For this review, take the finished solid that the model builds, in its own axes (mm). Face numbers are marked on the shaded views. A direction names the side the tool comes from. Coordinates: 2 decimals unless noted, no trailing zeros. Order: outer loops, then holes, each group sorted by start corner. A loop starts at its lowest first (then second) coordinate and runs counter-clockwise, first axis right, second up.
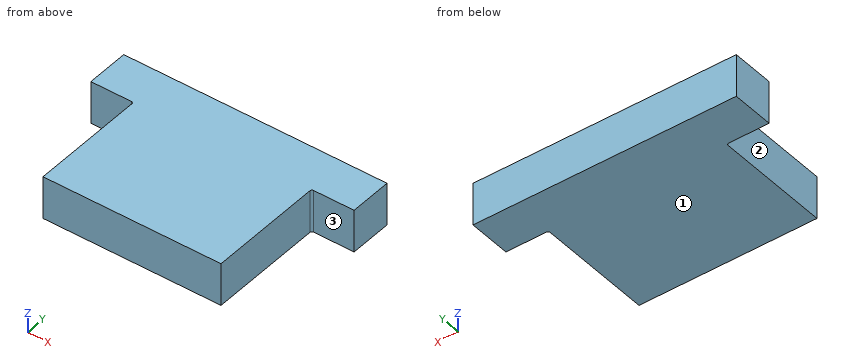
Autodesk Inventor part; units mm, degrees
ref_plane "YZ Plane" through (0, 0, 0) normal (1, 0, 0) x (0, 1, 0)
ref_plane "XZ Plane" through (0, 0, 0) normal (0, 1, 0) x (-1, 0, 0)
ref_plane "XY Plane" through (0, 0, 0) normal (0, 0, 1) x (1, 0, 0)
sketch "Sketch1" plane through (0, 0, 0) normal (0, 0, 1) x (1, 0, 0)
  line L0 (4.175, -3.75) -> (-4.175, -3.75)
  line L1 (-4.175, -3.75) -> (-4.175, 3.75)
  line L2 (-4.175, 3.75) -> (4.175, 3.75)
  line L3 (4.175, 3.75) -> (4.175, -3.75)
  line L4 (4.175, -3.75) -> (-4.175, 3.75) construction
  line L5 (-4.175, -3.75) -> (4.175, 3.75) construction
  point P0 (0, 0)
  dimension "d0" = 8.35
  dimension "d1" = 7.5
extrude "Extrusion1" add sketch "Sketch1" along normal mid plane 2
sketch "Sketch2" plane through (4.175, -3.75, 1) normal (1, 0, 0) x (0, 0, -1)
  line L0 (2, 7.5) -> (0, 7.5)
  line L1 (2, 7.5) -> (0, 7.5)
  line L2 (0, 7.5) -> (0, 5.5)
  line L3 (0, 5.5) -> (2, 5.5)
  line L4 (2, 5.5) -> (2, 7.5)
  point P0 (1, 3.75)
  dimension "d4" = 2
  dimension "d5" = 2
extrude "Extrusion2" add sketch "Sketch2" along normal blind 2
sketch "Sketch3" plane through (-4.175, -3.75, 1) normal (-1, 0, 0) x (0, 0, 1)
  line L0 (-2, 7.5) -> (0, 7.5)
  line L1 (0, 7.5) -> (0, 0)
  line L2 (-2, 7.5) -> (0, 7.5)
  line L3 (0, 7.5) -> (0, 5.5)
  line L4 (0, 5.5) -> (-2, 5.5)
  line L5 (-2, 5.5) -> (-2, 7.5)
  point P0 (-1, 3.75)
  dimension "d8" = 2
extrude "Extrusion3" add sketch "Sketch3" along normal blind 2
fillet "Fillet1" radius 0.1 2 edges at (4.175, 1.75, 0) (-4.175, 1.75, 0)
properties part number "Tapa_2_TFM"
1. Clearance check with flat-ended pins moving along their axes: pin 1 Ø0.9 at (x, z) = (5.5, 0) entering from -Y; pin 2 Ø1 at (y, z) = (-1, 0) entering from -X (3 decimals). State where each tip first meets the part, or that it passes through.
Answer below:
pin 1: stops at y = 1.75
pin 2: stops at x = -4.175
2. Machinability: for the marked faces 1, 2 and 3, which of the approach directions +Z, -Z, +X, -X, +Y, -Y give a long, thin tool a straight path to every point of the face, cutting with its end or side? Answer none if there is none.
Answer below:
face 1: -Z, +X, -X, +Y, -Y
face 2: +Z, -Z, -X, -Y
face 3: +Z, -Z, +X, -Y
3. To check wall thickness, follow L1, parallel to Y at x = 4.5, z = 0.5; L2, parallel to X at y = -2.5, z = -0.6 (3 decimals). State the ranges of each line that lie inside material, in increasing order.
Answer below:
L1: y = 1.75 to 3.75
L2: x = -4.175 to 4.175
4. Take a section at A-A, the plane z = 0.75. Give the boundary of the cut face in (x, y) (3 decimals), plus the area to 3 significant figures.
Answer below:
outline: (-6.175, 1.75) - (-4.275, 1.75) arc R0.1 cw to (-4.175, 1.65) - (-4.175, -3.75) - (4.175, -3.75) - (4.175, 1.65) arc R0.1 cw to (4.275, 1.75) - (6.175, 1.75) - (6.175, 3.75) - (-6.175, 3.75) - close
area: 70.6 mm2
5. Take a section at C-C, the plane y = 0.75. Give the boundary of the cut face in (x, z) (3 decimals).
Answer below:
outline: (-4.175, -1) - (4.175, -1) - (4.175, 1) - (-4.175, 1) - close
6. Take a section at B-B, the plane x = 5. Give the boundary of the cut face in (y, z).
Answer below:
outline: (1.75, -1) - (3.75, -1) - (3.75, 1) - (1.75, 1) - close
